Input: dimensioned drawing with shaded views. Units: mm. Origin: part minimum x, y, z. A direction names the side the tool comes from. Round coordinates to 2 decimals unless told otherwise and drop trailing zeros. Loops run counter-clockwise (first coordinate to the right, second up) from the corner with the lowest first, then second, coordinate; pieces in that order, holes last. Notation, with made-up numbers: M -29,86.25 L -8,86.25 A25 ccw -8,111.25 Z; hole C 89,-4 d6. An arc over 180 degrees is marked long. Put each result on its own line as item: value. Start each with the question number.
1) Section C-C on z = 238.5. Output: boundary loops of the cut face in (x, y) (1 decimal), plus the area to 3 significant figures.
2) Section A-A on x = 81.5. Output: boundary loops of the cut face in (y, z), plus the area to 3 significant figures.
3) Line query: probe 1 along Z at (x, y) = (66.5, 633); probe 2 along Y at (x, z) = (101.5, 631). Output: solid intervals per line, ascending.
4) Pin query (flat end, axial travel): pin 1 (2 mm diameter, centred on x = 395.5, y = 674, fed in from +Z); pin 2 (12 mm diameter, centred on x = 820, z = 389.5, fed in from -Y). Return the tip coordinate at first contact, or that it passes through.
5) Section B-B on y = 327. Output: boundary loops of the cut face in (x, z).
6) Section D-D on x = 695.5. Output: boundary loops of the cut face in (y, z).
7) Reachability of the marked faces 1, 2 and 3 from +Z, -Z, +X, -X, +Y, -Y: full face, straight path, thin tool, end or side. Return the list, or none.
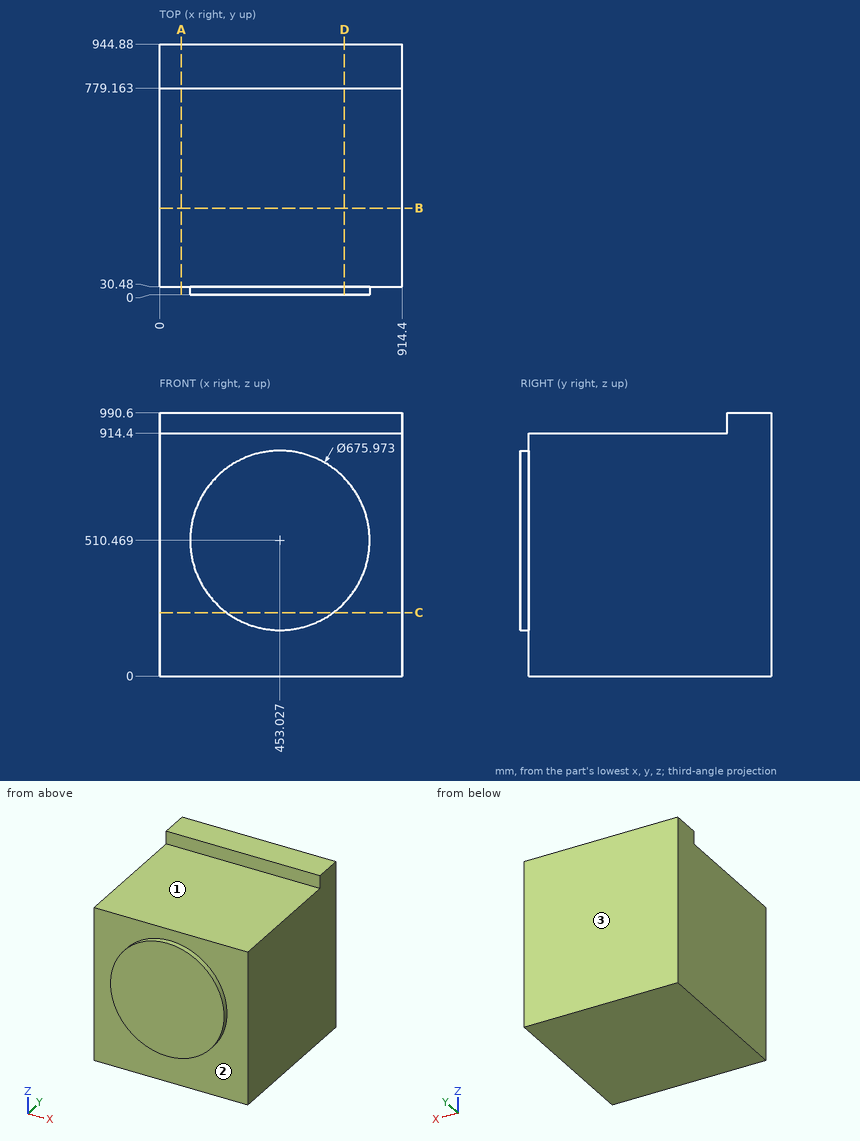
Geometry results:
1. outline: M 0,30.5 L 252.4,30.5 L 252.4,0 L 653.7,0 L 653.7,30.5 L 914.4,30.5 L 914.4,944.9 L 0,944.9 Z
1. area: 848,000 mm²
2. outline: M 30.48,0 L 944.88,0 L 944.88,990.6 L 779.16,990.6 L 779.16,914.4 L 30.48,914.4 Z
2. area: 849,000 mm²
3. probe 1: z = 0 to 914.4
3. probe 2: y = 30.48 to 944.88
4. pin 1: stops at z = 914.4
4. pin 2: stops at y = 30.48
5. outline: M 0,0 L 914.4,0 L 914.4,914.4 L 0,914.4 Z
6. outline: M 0,275.01 L 30.48,275.01 L 30.48,0 L 944.88,0 L 944.88,990.6 L 779.16,990.6 L 779.16,914.4 L 30.48,914.4 L 30.48,745.93 L 0,745.93 Z
7. face 1: +Z, +X, -X, -Y
7. face 2: -Y
7. face 3: +Z, -Z, +X, -X, +Y
